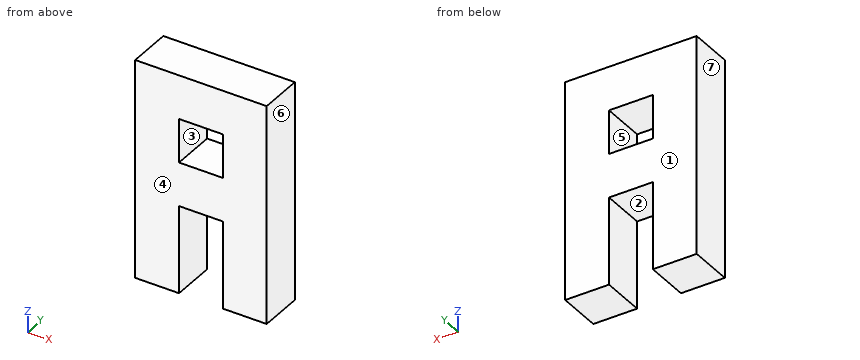
from build123d import *

# Parameters (mm, degrees)
F0_W     = 76.2
F0_H     = 127
F1_DEPTH = 25.4
F2_W     = 25.4
F2_H     = 50.8
F3_DEPTH = 25.401
F4_W     = 25.4
F4_H     = 25.4
F5_DEPTH = 25.401


with BuildPart() as f1:
    # F0 (on Front) → F1 (new body)
    with BuildSketch(Plane.XZ):
        Rectangle(F0_W, F0_H)
    extrude(amount=F1_DEPTH)

    # F2 (on face) → F3 (cut, through all)
    with BuildSketch(Plane.XZ.offset(25.4)):
        with Locations((0, -38.1)):
            Rectangle(F2_W, F2_H)
    extrude(amount=-F3_DEPTH, mode=Mode.SUBTRACT)

    # F4 (on face) → F5 (cut, through all)
    with BuildSketch(Plane.XZ.offset(25.4)):
        with Locations((0, 25.4)):
            Rectangle(F4_W, F4_H)
    extrude(amount=-F5_DEPTH, mode=Mode.SUBTRACT)


solid = f1.part
Work out the finished part from the listing and answer in its coordinate system (mm). Face numbers are marked on the shaded views. A direction names the side the tool comes from. Round coordinates to 2 decimals unless told otherwise and drop trailing zeros. Loops run counter-clockwise (first coordinate to the right, second up) from the corner with the lowest first, then second, coordinate; pieces in that order, holes last. Notation, with made-up numbers: M -25,47 L 5,47 A25 ccw 5,59 Z; hole C 32.5,87 d3. An arc over 180 degrees is marked long. One line per question, with ' | ' between items. Start each with the question number.
(1) A tool of negligible diameter and unlimited length cuts with its end or side. For the marked faces 1, 2 and 3, from which of +Z, -Z, +X, -X, +Y, -Y can it reach the whole face along a straight path? Write none if from no direction.
(2) A cutting plane is placed at C-C on x = -1. Write down the section's boundary in (y, z).
(3) For a pull along X with two mould halves and no side action, classify the marked faces 4, 5, 6 and 7 as released by +X, released by -X, zero draft, split by the parting line, or undercut.
(4) Find the intervals of material crossed by line 1 (X direction, y = -19, z = -29.5); line 2 (Z direction, x = 3, y = -11.75), in increasing order.
(5) A cutting plane is placed at B-B on y = -12.5. Write down the section's boundary in (x, z).
(6) A cutting plane is placed at A-A on z = 27. Write down the section's boundary in (x, y).
(7) Flat-ended cylindrical pins translate along their axes: pin 1 Ø2 at (x, z) = (30, 1) entering from +Y; pin 2 Ø7.5 at (x, y) = (2, -12.5) entering from -Z. Find the tip coordinate at first contact, or state that the pin passes through.
Geometry check:
1) face 1: +Z, -Z, +X, -X, +Y | face 2: -Z, +Y, -Y | face 3: +Y, -Y
2) outline: M -25.4,-12.7 L 0,-12.7 L 0,12.7 L -25.4,12.7 Z; M -25.4,38.1 L 0,38.1 L 0,63.5 L -25.4,63.5 Z
3) face 4: zero draft | face 5: undercut | face 6: released by +X | face 7: released by -X
4) line 1: x = -38.1 to -12.7, 12.7 to 38.1 | line 2: z = -12.7 to 12.7, 38.1 to 63.5
5) outline: M -38.1,-63.5 L -12.7,-63.5 L -12.7,-12.7 L 12.7,-12.7 L 12.7,-63.5 L 38.1,-63.5 L 38.1,63.5 L -38.1,63.5 Z; hole M -12.7,12.7 L 12.7,12.7 L 12.7,38.1 L -12.7,38.1 Z
6) outline: M -38.1,-25.4 L -12.7,-25.4 L -12.7,0 L -38.1,0 Z; M 12.7,-25.4 L 38.1,-25.4 L 38.1,0 L 12.7,0 Z
7) pin 1: stops at y = 0 | pin 2: stops at z = -12.7
